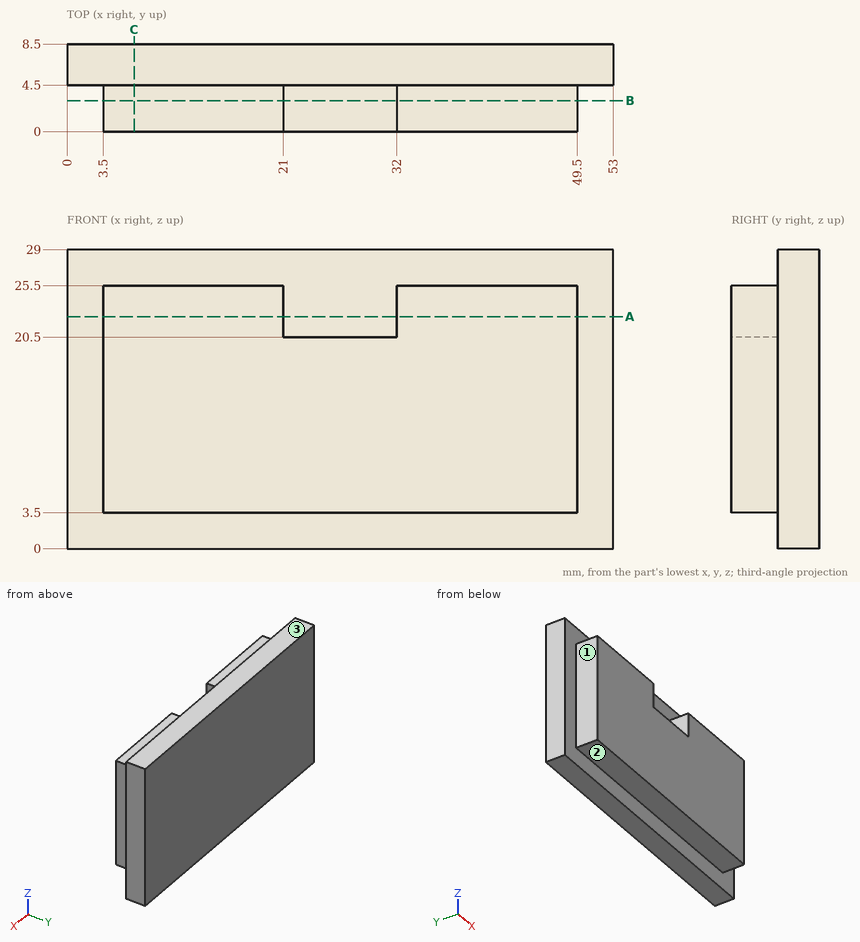
Here's the drawing with two shaded views (mm, measured from the low corner). I have some questions. A direction names the side the tool comes from. Give positions to 0.01 mm unless a question says otherwise; leave off trailing zeros. Order: outer loops, then holes, each group sorted by start corner. A loop starts at its lowest first (then second) coordinate and runs counter-clockwise, first axis right, second up. Notation, with made-up numbers: M -34.5,64 L 18.5,64 A13 ccw 18.5,78 Z; hole C -16.5,51 d1. An arc over 180 degrees is marked long. One line per item, written item: value.
1) For P1, Ø2, axis at x = 36, y = 3, coming from the -Z side; P2, Ø5, axis at x = 16, y = 1.5, coming from the +Z side; P3, Ø1.3, axis at y = 2.5, z = 10, coming from the +X side, each with a flat end and sliding along its axis, tell me the tip position at first contact or that it passes through.
Answer sheet:
P1: stops at z = 3.5
P2: stops at z = 25.5
P3: stops at x = 49.5
2) I want a section at B-B, the plane y = 3. List the corners of the cut face in (x, z) for me.
Answer sheet:
outline: M 3.5,3.5 L 49.5,3.5 L 49.5,25.5 L 32,25.5 L 32,20.5 L 21,20.5 L 21,25.5 L 3.5,25.5 Z
3) On a 3-axis mill with a long thin cutter (end or side, diameter ignored), from which of +Z, -Z, +X, -X, +Y, -Y can I reach the whole of each face in a straight line? I mean the marked faces 1, 2 and 3. Say none if no direction works.
Answer sheet:
face 1: +Z, -Z, -X, -Y
face 2: -Z, +X, -X, -Y
face 3: +Z, +X, -X, +Y, -Y
4) Please list where these lines run through material, in increasing order: line 1 along X through (y, z) = (3, 24.25); line 2 along X through (y, z) = (1.5, 8.75); line 3 along Y through (x, z) = (31, 2).
Answer sheet:
line 1: x = 3.5 to 21, 32 to 49.5
line 2: x = 3.5 to 49.5
line 3: y = 4.5 to 8.5
5) I want a section at A-A, the plane z = 22.5. List the corners of the cut face in (x, y) for me, plus the area to 4 significant figures.
Answer sheet:
outline: M 0,4.5 L 3.5,4.5 L 3.5,0 L 21,0 L 21,4.5 L 32,4.5 L 32,0 L 49.5,0 L 49.5,4.5 L 53,4.5 L 53,8.5 L 0,8.5 Z
area: 369.5 mm^2
6) I want a section at C-C, the plane x = 6.5. List the corners of the cut face in (y, z) for me, plus the area to 3 significant figures.
Answer sheet:
outline: M 0,3.5 L 4.5,3.5 L 4.5,0 L 8.5,0 L 8.5,29 L 4.5,29 L 4.5,25.5 L 0,25.5 Z
area: 215 mm^2
